```python
from build123d import *

# Parameters (mm, degrees)
F1_DEPTH = 3
F2_SIZE  = 1
F3_SIZE  = 1
F4_SIZE  = 1
F5_SIZE  = 1
F6_SIZE  = 1
F7_R     = 1.425
F8_DEPTH = 3.001
F9_R     = 5
F10_R    = 5
F11_R    = 5
F12_R    = 5
F13_R    = 5
F14_R    = 5
F15_R    = 5
F16_R    = 5


with BuildPart() as f1:
    # F0 (on Front) → F1 (new body)
    with BuildSketch(Plane.XZ):
        with BuildLine():
            ThreePointArc((10.8166538264, 2), (10.9540675571, 1.004193186), (11, 0))
            ThreePointArc((11, 0), (10.9540675571, -1.004193186), (10.8166538264, -2))
            Line((10.8166538264, -2), (14.8660687473, -2))
            ThreePointArc((14.8660687473, -2), (14.9664797332, -1.0022396895), (15, 0))
            ThreePointArc((15, 0), (14.9664797332, 1.0022396895), (14.8660687473, 2))
            Line((14.8660687473, 2), (10.8166538264, 2))
        make_face()
        with BuildLine():
            ThreePointArc((2, 10.8166538264), (7.7781745931, 7.7781745931), (10.8166538264, 2))
            Line((10.8166538264, 2), (14.8660687473, 2))
            ThreePointArc((14.8660687473, 2), (10.6066017178, 10.6066017178), (2, 14.8660687473))
            Line((2, 14.8660687473), (2, 10.8166538264))
        make_face()
        with BuildLine():
            Line((14.8660687473, -2), (10.8166538264, -2))
            ThreePointArc((10.8166538264, -2), (7.7781745931, -7.7781745931), (2, -10.8166538264))
            Line((2, -10.8166538264), (2, -14.8660687473))
            ThreePointArc((2, -14.8660687473), (10.6066017178, -10.6066017178), (14.8660687473, -2))
        make_face()
        with BuildLine():
            ThreePointArc((-2, 10.8166538264), (0, 11), (2, 10.8166538264))
            Line((2, 10.8166538264), (2, 14.8660687473))
            ThreePointArc((2, 14.8660687473), (0, 15), (-2, 14.8660687473))
            Line((-2, 14.8660687473), (-2, 10.8166538264))
        make_face()
        with BuildLine():
            Line((21, 2), (14.8660687473, 2))
            ThreePointArc((14.8660687473, 2), (14.9664797332, 1.0022396895), (15, 0))
            ThreePointArc((15, 0), (14.9664797332, -1.0022396895), (14.8660687473, -2))
            Line((14.8660687473, -2), (21, -2))
            Line((21, -2), (21, 2))
        make_face()
        with BuildLine():
            Line((2, -14.8660687473), (2, -10.8166538264))
            ThreePointArc((2, -10.8166538264), (0, -11), (-2, -10.8166538264))
            Line((-2, -10.8166538264), (-2, -14.8660687473))
            ThreePointArc((-2, -14.8660687473), (0, -15), (2, -14.8660687473))
        make_face()
        with BuildLine():
            ThreePointArc((-10.8166538264, 2), (-7.7781745931, 7.7781745931), (-2, 10.8166538264))
            Line((-2, 10.8166538264), (-2, 14.8660687473))
            ThreePointArc((-2, 14.8660687473), (-10.6066017178, 10.6066017178), (-14.8660687473, 2))
            Line((-14.8660687473, 2), (-10.8166538264, 2))
        make_face()
        with BuildLine():
            ThreePointArc((-2, 14.8660687473), (0, 15), (2, 14.8660687473))
            Line((2, 14.8660687473), (2, 21))
            Line((2, 21), (-2, 21))
            Line((-2, 21), (-2, 14.8660687473))
        make_face()
        with BuildLine():
            Line((-2, -14.8660687473), (-2, -10.8166538264))
            ThreePointArc((-2, -10.8166538264), (-7.7781745931, -7.7781745931), (-10.8166538264, -2))
            Line((-10.8166538264, -2), (-14.8660687473, -2))
            ThreePointArc((-14.8660687473, -2), (-10.6066017178, -10.6066017178), (-2, -14.8660687473))
        make_face()
        with BuildLine():
            Line((2, -21), (2, -14.8660687473))
            ThreePointArc((2, -14.8660687473), (0, -15), (-2, -14.8660687473))
            Line((-2, -14.8660687473), (-2, -21))
            Line((-2, -21), (2, -21))
        make_face()
        with BuildLine():
            ThreePointArc((-10.8166538264, -2), (-11, 0), (-10.8166538264, 2))
            Line((-10.8166538264, 2), (-14.8660687473, 2))
            ThreePointArc((-14.8660687473, 2), (-15, 0), (-14.8660687473, -2))
            Line((-14.8660687473, -2), (-10.8166538264, -2))
        make_face()
        with BuildLine():
            ThreePointArc((-14.8660687473, -2), (-15, 0), (-14.8660687473, 2))
            Line((-14.8660687473, 2), (-21, 2))
            Line((-21, 2), (-21, -2))
            Line((-21, -2), (-14.8660687473, -2))
        make_face()
    extrude(amount=F1_DEPTH)

    # F2
    f2_edges = [f1.edges().sort_by_distance(p)[0] for p in [
        (-2, -1.5, 21),
    ]]
    chamfer(f2_edges, length=F2_SIZE)

    # F3
    f3_edges = [f1.edges().sort_by_distance(p)[0] for p in [
        (2, -1.5, 21),
    ]]
    chamfer(f3_edges, length=F3_SIZE)

    # F4
    f4_edges = [f1.edges().sort_by_distance(p)[0] for p in [
        (21, -1.5, 2),
        (21, -1.5, -2),
    ]]
    chamfer(f4_edges, length=F4_SIZE)

    # F5
    f5_edges = [f1.edges().sort_by_distance(p)[0] for p in [
        (2, -1.5, -21),
        (-2, -1.5, -21),
    ]]
    chamfer(f5_edges, length=F5_SIZE)

    # F6
    f6_edges = [f1.edges().sort_by_distance(p)[0] for p in [
        (-21, -1.5, 2),
        (-21, -1.5, -2),
    ]]
    chamfer(f6_edges, length=F6_SIZE)

    # F7 (on Front) → F8 (cut, through all)
    with BuildSketch(Plane.XZ):
        with Locations((0, 15)):
            Circle(F7_R)
        with Locations((15, 0)):
            Circle(F7_R)
        with Locations((-15, 0)):
            Circle(F7_R)
        with Locations((0, -15)):
            Circle(F7_R)
    extrude(amount=F8_DEPTH, mode=Mode.SUBTRACT)

    # F9
    f9_edges = [f1.edges().sort_by_distance(p)[0] for p in [
        (-2, -1.5, 14.866069),
    ]]
    fillet(f9_edges, radius=F9_R)

    # F10
    f10_edges = [f1.edges().sort_by_distance(p)[0] for p in [
        (2, -1.5, 14.866069),
    ]]
    fillet(f10_edges, radius=F10_R)

    # F11
    f11_edges = [f1.edges().sort_by_distance(p)[0] for p in [
        (14.866069, -1.5, -2),
    ]]
    fillet(f11_edges, radius=F11_R)

    # F12
    f12_edges = [f1.edges().sort_by_distance(p)[0] for p in [
        (-2, -1.5, -14.866069),
    ]]
    fillet(f12_edges, radius=F12_R)

    # F13
    f13_edges = [f1.edges().sort_by_distance(p)[0] for p in [
        (2, -1.5, -14.866069),
    ]]
    fillet(f13_edges, radius=F13_R)

    # F14
    f14_edges = [f1.edges().sort_by_distance(p)[0] for p in [
        (14.866069, -1.5, 2),
    ]]
    fillet(f14_edges, radius=F14_R)

    # F15
    f15_edges = [f1.edges().sort_by_distance(p)[0] for p in [
        (-14.866069, -1.5, -2),
    ]]
    fillet(f15_edges, radius=F15_R)

    # F16
    f16_edges = [f1.edges().sort_by_distance(p)[0] for p in [
        (-14.866069, -1.5, 2),
    ]]
    fillet(f16_edges, radius=F16_R)


solid = f1.part
```
The model under review builds one solid part; all positions refer to its coordinate system, in mm. A direction names the side the tool comes from. Round coordinates to 2 decimals unless told otherwise and drop trailing zeros. Loops run counter-clockwise (first coordinate to the right, second up) from the corner with the lowest first, then second, coordinate; pieces in that order, holes last. Notation, with made-up numbers: (25, 72.25) - (29, 72.25) arc R14 ccw to (29, 83.25) - close; hole circle Ø11 at (37.5, -30). An arc over 180 degrees is marked (long way). Use a Markdown table: item, result. Add a question column.
Q1. Add section A-A (z = -6). State the section outline as (x, y) points.
Q2. Machinability: for faces 1 (the face through (-2, -1, 19)), 2 (the face through (19, -1, 2)), 3 (the face through (-2, -1, -19)), which of the approach directions +Z, -Z, +X, -X, +Y, -Y give a long, thin tool a straight path to every point of the face, cutting with its end or side? Answer none if there is none.
Q3. Add section B-B (x = -15). State the section outline as (y, z) points (3 decimals).
Q4. Add section C-C (y = -2.2). State how many separate pieces and enclosed holes the cut face has, plus the area to 3 significant figures.
Q5. For probe 1 along Z at (x, y) = (0, -1.65) (3 decimals); probe 2 along Z at (x, y) = (-2.5, -0.85), list the stretches that pass through material, from the lowest coordinate up.
Q6. The part is to be moulded in two halves that separate along X. For faces 4 (the face through (-13.684, -1.479, -0.546)), 5 (the face through (-15.92, -1.52, 2.87)), 6 (the face through (-19, -1, 2)), say which applies: pulls with the +X half, pulls with the -X half, needs draft (parallel to the pull), parting line crosses it, or undercut.
Q7. Insertion check: pin 1 Ø1 at (y, z) = (-1, 19.5) entering from +X; pin 2 Ø0.6 at (x, y) = (19.5, -1.5) entering from +Z; pin 3 Ø1 at (x, z) = (14, -5) entering from +Y; pin 4 Ø0.6 at (x, y) = (19, -2) entering from -Z. Each pin has a flat end and moves straight along its axis. Give the tip position at first contact, or say it passes through.
Worked answers:
| question | item | result |
|---|---|---|
| 1 | outline | (-13.75, -3) - (-9.22, -3) - (-9.22, 0) - (-13.75, 0) - close; (9.22, -3) - (13.75, -3) - (13.75, 0) - (9.22, 0) - close |
| 2 | face 1 | +Z, -X, +Y, -Y |
| 2 | face 2 | +Z, +X, +Y, -Y |
| 2 | face 3 | -Z, -X, +Y, -Y |
| 3 | outline | (-3, -3.676) - (0, -3.676) - (0, -1.425) - (-3, -1.425) - close; (-3, 1.425) - (0, 1.425) - (0, 3.676) - (-3, 3.676) - close |
| 4 | separate pieces | 1 |
| 4 | enclosed holes | 5 |
| 4 | area | 415 mm² |
| 5 | probe 1 | -21 to -16.425, -13.575 to -11, 11 to 13.575, 16.425 to 21 |
| 5 | probe 2 | -16.56 to -10.71, 10.71 to 16.56 |
| 6 | face 4 | undercut |
| 6 | face 5 | pulls with the -X half |
| 6 | face 6 | needs draft |
| 7 | pin 1 | x = 2 |
| 7 | pin 2 | z = 2 |
| 7 | pin 3 | y = 0 |
| 7 | pin 4 | z = -2 |
